Verification items for the finished model (mm, model axes). A direction names the side the tool comes from. Coordinates: 2 decimals unless noted, no trailing zeros. Loops run counter-clockwise (first coordinate to the right, second up) from the corner with the lowest first, then second, coordinate; pieces in that order, holes last. Notation, with made-up numbers: (12.5, -12.5) -> (28.5, -12.5) arc R27 ccw to (28.5, 19.5) -> close; hole circle Ø11 at (23, -29). An arc over 180 degrees is marked (long way). Answer as a JSON object with one key per item and string values. Group by question number.
Q1. Cross-section at C-C on z = -2. Record the boundary of the cut face in (x, y), and give its area (4 significant figures).
Q2. Gauge pin test, flat ends, axial feed: pin 1 Ø1.1 at (x, z) = (1.5, -2) entering from -Y; pin 2 Ø1.8 at (y, z) = (0, -2.5) entering from -X; pin 3 Ø1.3 at (y, z) = (-0.5, 3) entering from -X. Record the tip position at first contact, or that the pin passes through.
Q3. Cross-section at B-B on y = -2. Record the boundary of the cut face in (x, z), and give its area (4 significant figures).
Q4. Scan lines: L1, parallel to X at y = 0.25, z = 3.25; L2, parallel to Z at x = 7, y = 2.35; L3, parallel to Z at x = -3.5, y = 1.5. Record each from-to range of solid material in increasing order.
Q5. Cross-section at A-A on x = 0.25. Record the boundary of the cut face in (y, z), and give its area (3 significant figures).
Q6. Cross-section at D-D on y = 1.4. Record the boundary of the cut face in (x, z).
Q7. Set-up check for faces 1 (the flat face through (-5.25, 0, 3)), 2 (the flat face through (-3.25, 0, -2)), 3 (the flat face through (0, 1.75, -2)), 4 (the flat face through (5.25, 0, 3)): record each of +Z, -Z, +X, -X, +Y, -Y from which the full face is reachable in a straight line by a thin tool's end or side.
```python
from build123d import *

# Parameters (mm, degrees)
F0_W     = 20
F0_H     = 5.5
F1_DEPTH = 0.5
F2_W     = 10.5
F2_H     = 5.5
F3_DEPTH = 4.5
F4_W     = 6.5
F4_H     = 3.5
F5_DEPTH = 3.8


with BuildPart() as f1:
    # F0 (on Top) → F1 (new body)
    with BuildSketch(Plane.XY):
        Rectangle(F0_W, F0_H)
    extrude(amount=F1_DEPTH)

    # F2 (on face) → F3 (join)
    with BuildSketch(Plane.XY.offset(0.5)):
        Rectangle(F2_W, F2_H)
    extrude(amount=F3_DEPTH)

    # F4 (on face) → F5 (join)
    with BuildSketch(Plane(origin=(0, 0, 0), x_dir=(1, 0, 0), z_dir=(0, 0, -1))):
        Rectangle(F4_W, F4_H)
    extrude(amount=F5_DEPTH)


solid = f1.part
```
Computed values:
{
 "1": {"outline": "(-3.25, -1.75) -> (3.25, -1.75) -> (3.25, 1.75) -> (-3.25, 1.75) -> close", "area": "22.75 mm²"},
 "2": {"pin 1": "stops at y = -1.75", "pin 2": "stops at x = -3.25", "pin 3": "stops at x = -5.25"},
 "3": {"outline": "(-10, 0) -> (10, 0) -> (10, 0.5) -> (5.25, 0.5) -> (5.25, 5) -> (-5.25, 5) -> (-5.25, 0.5) -> (-10, 0.5) -> close", "area": "57.25 mm²"},
 "4": {"L1": "x = -5.25 to 5.25", "L2": "z = 0 to 0.5", "L3": "z = 0 to 5"},
 "5": {"outline": "(-2.75, 0) -> (-1.75, 0) -> (-1.75, -3.8) -> (1.75, -3.8) -> (1.75, 0) -> (2.75, 0) -> (2.75, 5) -> (-2.75, 5) -> close", "area": "40.8 mm²"},
 "6": {"outline": "(-10, 0) -> (-3.25, 0) -> (-3.25, -3.8) -> (3.25, -3.8) -> (3.25, 0) -> (10, 0) -> (10, 0.5) -> (5.25, 0.5) -> (5.25, 5) -> (-5.25, 5) -> (-5.25, 0.5) -> (-10, 0.5) -> close"},
 "7": {"face 1": "+Z, -X, +Y, -Y", "face 2": "-Z, -X, +Y, -Y", "face 3": "-Z, +X, -X, +Y", "face 4": "+Z, +X, +Y, -Y"}
}
